Here's how the part is built. I have some questions about the finished solid (model axes, mm). Coordinates: 2 decimals unless noted, no trailing zeros. Write each loop counter-clockwise with the first axis right and the second up, starting at its lowest first coordinate (ties: lowest second). Pieces come first, ordered by that corner, then holes. Notation, with made-up numbers: M 59,80 L 85,80 A21 ccw 85,95 Z; hole C 51,44.25 d11. An arc over 180 degrees is marked long. Use a Markdown table: item, result.
Autodesk Inventor part; units mm, degrees
ref_plane "YZ Plane" through (0, 0, 0) normal (1, 0, 0) x (0, 1, 0)
ref_plane "XZ Plane" through (0, 0, 0) normal (0, 1, 0) x (-1, 0, 0)
ref_plane "XY Plane" through (0, 0, 0) normal (0, 0, 1) x (1, 0, 0)
sketch "Sketch1" plane through (0, 0, 0) normal (0, 1, 0) x (-1, 0, 0)
  line L0 (0, 0) -> (0, -160) construction
  line L1 (5, 0) -> (5, -160)
  line L2 (-5, -160) -> (-5, 0)
  arc A0 (5, 0) -> (-5, 0) centre (0, 0) ccw
  arc A1 (-5, -160) -> (5, -160) centre (0, -160) ccw
  circle A2 centre (0, 0) radius 1.65
  line L3 (0, -30) -> (0, -120) construction
  line L4 (1.65, -30) -> (1.65, -120)
  line L5 (-1.65, -120) -> (-1.65, -30)
  arc A3 (1.65, -30) -> (-1.65, -30) centre (0, -30) ccw
  arc A4 (-1.65, -120) -> (1.65, -120) centre (0, -120) ccw
  point P0 (0, -80)
  point P1 (0, -75)
  dimension "d0" = 160
  dimension "d1" = 10
  dimension "d2" = 3.3
  dimension "d3" = 30
  dimension "d5" = 120
  dimension "d6" = 3.3
extrude "Extrusion1" add sketch "Sketch1" along normal blind 6
sketch "Sketch2" plane through (5, 0, 0) normal (1, 0, 0) x (0, 0, -1)
  line L0 (160, 0) -> (160, 6)
  line L1 (0, 0) -> (160, 0)
  line L2 (160, 0) -> (160, 6)
  line L3 (0, 6) -> (160, 6)
  line L4 (0, 0) -> (0, 6)
  line L5 (160, 0) -> (160, 0)
  line L6 (160, 0) -> (160, 6)
  line L7 (160, 6) -> (160, 6)
  line L8 (160, 0) -> (160, 6)
  line L9 (160, 0) -> (0, 0)
  arc A0 (373.775, -84) -> (160, 0) centre (160, -314.0223) ccw
  line L10 (160, 6) -> (0, 6)
  arc A1 (373.775, -78) -> (160, 6) centre (160, -308.0223) ccw
  line L11 (373.775, -78) -> (373.775, -84)
  line L12 (0, 0) -> (160, 0)
  dimension "d9" = 6
  dimension "d10" = 373.775
  dimension "d11" = 90
extrude "Extrusion2" add sketch "Sketch2" against normal blind 10 contours L0 A1 L11 A0
fillet "Fillet1" radius 2 4 edges at (0, -78, -373.775) (5, -81, -373.775) (-5, -81, -373.775) (0, -84, -373.775)
sketch "Sketch3" plane through (0, 6, 0) normal (0, 1, 0) x (1, 0, 0)
  line L0 (36.6774, -16.9321) -> (-64.8889, -16.9321)
  line L1 (-64.8889, -16.9321) -> (-64.8889, 211.3912)
  line L2 (-64.8889, 211.3912) -> (36.6774, 211.3912)
  line L3 (36.6774, 211.3912) -> (36.6774, -16.9321)
  line L4 (-92.1247, 397.3107) -> (101.238, 397.3107)
  line L5 (101.238, 397.3107) -> (101.238, -55.9315)
  line L6 (101.238, -55.9315) -> (-92.1247, -55.9315)
  line L7 (-92.1247, -55.9315) -> (-92.1247, 397.3107)
  point P0 (0, 0)
extrude "Extrusion3" cut sketch "Sketch3" against normal blind 100 contours L0 L1 L2 L3
properties part number "Part_11_p1"
1. Suppose I cut it at C-C on z = -263. Write out the boundary of the cut face in (x, y).
Answers follow:
| item | result |
|---|---|
| outline | M -5,-17.37 L 5,-17.37 L 5,-11.37 L -5,-11.37 Z |
2. Will these pins go through, and if not, where does the flat tip stop? pin 1 Ø4 at (x, y) = (-3, -31) entering from -Z; pin 2 Ø3 at (x, z) = (4, -348) entering from -Y; pin 3 Ø2 at (x, y) = (-2, -19.5) entering from -Z.
Answers follow:
| item | result |
|---|---|
| pin 1 | stops at z = -311.57 |
| pin 2 | stops at y = -63.62 |
| pin 3 | stops at z = -286.26 |
3. Suppose I cut it at A-A on x = -1.25. Write out the boundary of the cut face in (y, z) (1 decimal), and give its area (3 significant figures).
Answers follow:
| item | result |
|---|---|
| outline | M -80.9,-370.4 A2 ccw -79.5,-373.8 L -78.9,-373.8 A2 ccw -77.4,-373.1 A314 ccw 1.8,-211.4 L -4.2,-211.4 A314 cw Z |
| area | 970 mm2 |
4. Suppose I cut it at B-B on y = -25.5. Write out the boundary of the cut face in (x, z), and give its area (3 significant figures).
Answers follow:
| item | result |
|---|---|
| outline | M -5,-297.08 L 5,-297.08 L 5,-283.96 L -5,-283.96 Z |
| area | 131 mm2 |
5. I need wall thicknesses on probe 1 along Y at (x, z) = (2.75, -247); probe 2 along Y at (x, z) = (2.5, -341); probe 3 along Z at (x, y) = (-1.25, -70). Which ranges of each line are inside material? Lowest first, please.
Answers follow:
| item | result |
|---|---|
| probe 1 | y = -12.29 to -6.29 |
| probe 2 | y = -57.41 to -51.41 |
| probe 3 | z = -364.83 to -357.64 |
